```python
from build123d import *

# Parameters (mm, degrees)
F1_DEPTH = 22.5
F2_R     = 2.5
F3_DEPTH = 5.001
F4_R     = 2.5
F5_DEPTH = 25


with BuildPart() as f1:
    # F0 (on Front) → F1 (new body)
    with BuildSketch(Plane.XZ):
        with BuildLine():
            Line((-28.054744, -5), (31.945256, -5))
            Line((31.945256, -5), (31.945256, 0))
            Line((31.945256, 0), (19.444446, 0))
            Line((19.444446, 0), (19.444446, 12.5))
            Line((19.444446, 12.5), (14.444446, 12.5))
            ThreePointArc((14.444446, 12.5), (1.944851, -0.100626), (-10.554744, 12.5))
            Line((-10.554744, 12.5), (-15.554744, 12.5))
            Line((-15.554744, 12.5), (-15.554744, 0))
            Line((-15.554744, 0), (-28.054744, 0))
            Line((-28.054744, 0), (-28.054744, -5))
        make_face()
    extrude(amount=F1_DEPTH)

    # F2 (on face) → F3 (cut, through all)
    with BuildSketch(Plane.XY):
        with Locations((23.958334, -11.25)):
            Circle(F2_R)
    extrude(amount=-F3_DEPTH, mode=Mode.SUBTRACT)

    # F4 (on face) → F5 (cut)
    with BuildSketch(Plane.XY):
        with Locations((-21.804744, -11.25)):
            Circle(F4_R)
    extrude(amount=-F5_DEPTH, mode=Mode.SUBTRACT)


solid = f1.part
```
The listing builds one solid part. Answer for the finished solid, in the listing's coordinates (mm). A direction names the side the tool comes from. Coordinates: 2 decimals unless noted, no trailing zeros. Loops run counter-clockwise (first coordinate to the right, second up) from the corner with the lowest first, then second, coordinate; pieces in that order, holes last. Notation, with made-up numbers: M 0.5,-4 L 35.5,-4 A32 cw 35.5,27 Z; hole C 51.5,53.5 d4. An arc over 180 degrees is marked long. Answer as a JSON object with one key per item and string values. Group by question number.
Item 1: Consider L1, parallel to X at y = -11, z = -2.75; L2, parallel to X at y = -3.5, z = 11; L3, parallel to Z at x = -20, y = -8. Determine where each line is inside the solid, lowest interval first.
Item 2: Section B-B (x = 23.5) is taken. Write down the section's boundary in (y, z), and give its area (3 significant figures).
Item 3: Determine the mould class of faces 1 (the face through (21.974, -12.771, -2.465)), 2 (the face through (-28.055, -11, -2)), 3 (the face through (2, -11, -5)) for opening direction X: +X half, -X half, draft (parallel to the pull), parting line (faces both ways), or undercut.
Item 4: Each of these flat-tipped pins is pushed along its axis until it touches: P1, Ø4, axis at y = -9, z = 7.5, coming from the +X side; P2, Ø1, axis at y = -2.5, z = 8, coming from the -X side. Where does it stop, or does it pass through?
Item 5: Which of the six approach directions +Z, -Z, +X, -X, +Y, -Y give full straight-line access (tool end or side, diameter ignored) to faces 4 (the face through (27, -11, 0)), 5 (the face through (-15.555, -11, 6)), 6 (the face through (-13, -11, 12.5))?
Item 6: Section C-C (z = 8.25) is taken. Write down the section's boundary in (x, y), and give its area (3 significant figures).
Solved:
{
 "1": {"L1": "x = -28.05 to -24.29, -19.32 to 21.47, 26.45 to 31.95", "L2": "x = -15.55 to -10.48, 14.37 to 19.44", "L3": "z = -5 to 0"},
 "2": {"outline": "M -22.5,-5 L -13.71,-5 L -13.71,0 L -22.5,0 Z; M -8.79,-5 L 0,-5 L 0,0 L -8.79,0 Z", "area": "87.9 mm2"},
 "3": {"face 1": "undercut", "face 2": "-X half", "face 3": "draft"},
 "4": {"P1": "stops at x = 19.44", "P2": "stops at x = -15.55"},
 "5": {"face 4": "+Z, +X, +Y, -Y", "face 5": "+Z, -X, +Y, -Y", "face 6": "+Z, +X, -X, +Y, -Y"},
 "6": {"outline": "M -15.55,-22.5 L -9.85,-22.5 L -9.85,0 L -15.55,0 Z; M 13.74,-22.5 L 19.44,-22.5 L 19.44,0 L 13.74,0 Z", "area": "257 mm2"}
}
